Work out the finished part from the listing and answer in its coordinate system (mm). Give positions to 0.01 mm unless a question says otherwise; leave off trailing zeros. Order: outer loops, then holes, each group sorted by start corner. A loop starts at its lowest first (then second) coordinate and runs counter-clockwise, first axis right, second up. Notation, with made-up numbers: (2, 72.5) -> (10, 72.5) arc R24 ccw to (10, 103.5) -> close; hole circle Ø3 at (71, -5). An arc over 180 degrees is marked (long way). Use a Markdown table: item, result. Add a question column.
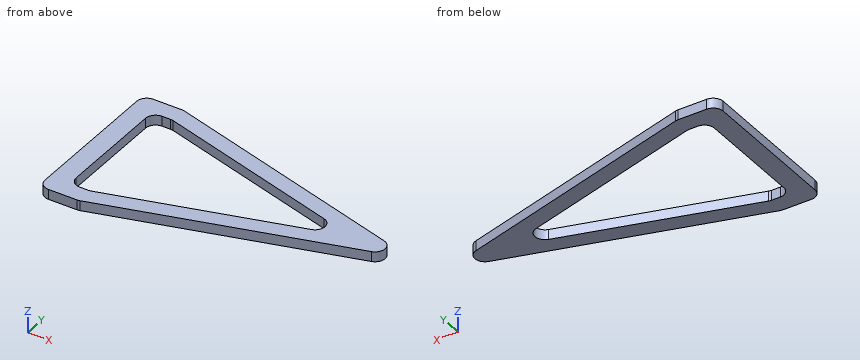
```python
from build123d import *

# Parameters (mm, degrees)
F1_DEPTH = 6.35
F2_W     = 12.7
F2_H     = 79.8285714286
F3_DEPTH = 6.35
F4_R     = 6.35
F5_R     = 6.35


with BuildPart() as f1:
    # F0 (on Top) → F1 (new body)
    with BuildSketch(Plane.XY):
        Polygon((-177.8, 0), (0, 0), (-177.8, 50.8), align=None)
        Polygon((-177.8, -50.8), (0, 0), (-177.8, 0), align=None)
        Polygon((-177.8, 0), (-177.8, 50.8), (-203.2, 50.8), (-203.2, -50.8), (-177.8, -50.8), align=None)
    extrude(amount=F1_DEPTH)

    # F2 (on face) → F3 (cut, through all)
    with BuildSketch(Plane.XY.offset(6.35)):
        Polygon((-177.8, 39.9142857143), (-177.8, -39.9142857143), (-38.1, 0), align=None)
        with Locations((-184.15, 0)):
            Rectangle(F2_W, F2_H)
    extrude(amount=-F3_DEPTH, mode=Mode.SUBTRACT)

    # F4
    f4_edges = [f1.edges().sort_by_distance(p)[0] for p in [
        (-177.8, -50.8, 3.175),
        (-177.8, 50.8, 3.175),
        (-203.2, -50.8, 3.175),
        (-203.2, 50.8, 3.175),
    ]]
    fillet(f4_edges, radius=F4_R)

    # F5
    f5_edges = [f1.edges().sort_by_distance(p)[0] for p in [
        (-177.8, -39.914286, 3.175),
        (-190.5, -39.914286, 3.175),
        (-190.5, 39.914286, 3.175),
        (-177.8, 39.914286, 3.175),
        (0, 0, 3.175),
        (-38.1, 0, 3.175),
    ]]
    fillet(f5_edges, radius=F5_R)


solid = f1.part
```
1) A flat-ended cylindrical pin translates along its axis: pin 1 (1 mm diameter, centred on x = -113.5, z = 4.5, fed in from -Y). Find the tip coordinate at first contact, or state that the pin passes through.
2) Straight lines are drawn through the part: line 1 (X direction, y = -3.5, z = 5.5); line 2 (Y direction, x = -75, z = 4.5); line 3 (Y direction, x = -104, z = 2.25). For each, find the intervals that lie inside material, in ascending order.
3) The part is cut by section C-C, the plane y = 3.5. Determine the outline of the cut face in (x, z).
4) The part is cut by section A-A, the plane z = 4.5. Determine the outline of the cut face in (x, y), then the cut area to 3 significant figures.
5) The part is cut by section D-D, the plane x = -47. Determine the outline of the cut face in (y, z).
6) The part is cut by section B-B, the plane x = -123. Determine the outline of the cut face in (y, z), then the cut area to 3 significant figures.
A:
| question | item | result |
|---|---|---|
| 1 | pin 1 | y = -32.57 |
| 2 | line 1 | -203.2 to -190.5, -55.92 to -17.82 |
| 2 | line 2 | -21.43 to -10.54, 10.54 to 21.43 |
| 2 | line 3 | -29.71 to -18.83, 18.83 to 29.71 |
| 3 | outline | (-203.2, 0) -> (-190.5, 0) -> (-190.5, 6.35) -> (-203.2, 6.35) -> close; (-55.92, 0) -> (-17.82, 0) -> (-17.82, 6.35) -> (-55.92, 6.35) -> close |
| 4 | outline | (-203.2, -44.45) arc R6.35 ccw to (-196.85, -50.8) -> (-178.69, -50.8) arc R6.35 ccw to (-176.94, -50.56) -> (-21.37, -6.11) arc R6.35 ccw to (-21.37, 6.11) -> (-176.94, 50.56) arc R6.35 ccw to (-178.69, 50.8) -> (-196.85, 50.8) arc R6.35 ccw to (-203.2, 44.45) -> close; hole (-190.5, -33.56) arc R6.35 ccw to (-184.15, -39.91) -> (-178.69, -39.91) arc R6.35 ccw to (-176.94, -39.67) -> (-59.47, -6.11) arc R6.35 ccw to (-59.47, 6.11) -> (-176.94, 39.67) arc R6.35 ccw to (-178.69, 39.91) -> (-184.15, 39.91) arc R6.35 ccw to (-190.5, 33.56) -> close |
| 4 | area | 5,020 mm^2 |
| 5 | outline | (-13.43, 0) -> (13.43, 0) -> (13.43, 6.35) -> (-13.43, 6.35) -> close |
| 6 | outline | (-35.14, 0) -> (-24.26, 0) -> (-24.26, 6.35) -> (-35.14, 6.35) -> close; (24.26, 0) -> (35.14, 0) -> (35.14, 6.35) -> (24.26, 6.35) -> close |
| 6 | area | 138 mm^2 |
